from build123d import *

# Parameters (mm, degrees)
SKETCH1_R           = 12.5
SKETCH1_W           = 200
SKETCH1_H           = 15
BOSS_EXTRUDE1_DEPTH = 30
CUT_EXTRUDE2_REACH  = 204.793
SKETCH2_R           = 3.5
CUT_EXTRUDE3_START  = -27
SKETCH2_3_R         = 8
SKETCH2_3_R_2       = 3.5
CUT_EXTRUDE3_DEPTH  = 3
CUT_EXTRUDE4_REACH  = 204.793


with BuildPart() as part:
    # Sketch1 → Boss-Extrude1 (new body)
    with BuildSketch(Plane.XY):
        with Locations((175, 0)):
            Circle(SKETCH1_R)
        with Locations((100, 0)):
            Circle(SKETCH1_R)
        with Locations((100, 7.5)):
            Rectangle(SKETCH1_W, SKETCH1_H)
        with BuildLine():
            ThreePointArc((187.5, 0), (175, 12.5), (162.5, 0))
            Line((162.5, 0), (175, 0))
            Line((175, 0), (187.5, 0))
        make_face()
        with BuildLine():
            Line((175, 0), (162.5, 0))
            ThreePointArc((162.5, 0), (175, -12.5), (187.5, 0))
            Line((187.5, 0), (175, 0))
        make_face()
        with BuildLine():
            ThreePointArc((187.5, 0), (175, 12.5), (162.5, 0))
            Line((162.5, 0), (175, 0))
            Line((175, 0), (187.5, 0))
        make_face()
        with BuildLine():
            Line((175, 0), (162.5, 0))
            ThreePointArc((162.5, 0), (175, -12.5), (187.5, 0))
            Line((187.5, 0), (175, 0))
        make_face()
        with BuildLine():
            ThreePointArc((112.5, 0), (100, 12.5), (87.5, 0))
            Line((87.5, 0), (100, 0))
            Line((100, 0), (112.5, 0))
        make_face()
        with BuildLine():
            Line((100, 0), (87.5, 0))
            ThreePointArc((87.5, 0), (100, -12.5), (112.5, 0))
            Line((112.5, 0), (100, 0))
        make_face()
        with BuildLine():
            ThreePointArc((112.5, 0), (100, 12.5), (87.5, 0))
            Line((87.5, 0), (100, 0))
            Line((100, 0), (112.5, 0))
        make_face()
        with BuildLine():
            Line((100, 0), (87.5, 0))
            ThreePointArc((87.5, 0), (100, -12.5), (112.5, 0))
            Line((112.5, 0), (100, 0))
        make_face()
    extrude(amount=BOSS_EXTRUDE1_DEPTH)

    # Sketch2 → Cut-Extrude2 (cut, up to next)
    with BuildSketch(Plane.XY.offset(30), mode=Mode.PRIVATE) as cut_extrude2_sk1:
        with Locations((100, 0)):
            Circle(SKETCH2_R)
    cut_extrude2_tool1 = extrude(cut_extrude2_sk1.sketch, amount=-CUT_EXTRUDE2_REACH, mode=Mode.PRIVATE) & part.part
    # Sketch2 → Cut-Extrude2 (cut, up to next)
    with BuildSketch(Plane.XY.offset(30), mode=Mode.PRIVATE) as cut_extrude2_sk2:
        with Locations((175, 0)):
            Circle(SKETCH2_R)
    cut_extrude2_tool2 = extrude(cut_extrude2_sk2.sketch, amount=-CUT_EXTRUDE2_REACH, mode=Mode.PRIVATE) & part.part
    add(cut_extrude2_tool1.solids().sort_by_distance((100, 0, 30))[0], mode=Mode.SUBTRACT)
    add(cut_extrude2_tool2.solids().sort_by_distance((175, 0, 30))[0], mode=Mode.SUBTRACT)

    # Sketch2<3> → Cut-Extrude3 (cut)
    # profile 1 of 2: a face of its own
    with BuildSketch(Plane.XY.offset(30).offset(CUT_EXTRUDE3_START)):
        with Locations((100, 0)):
            Circle(SKETCH2_3_R)
        with Locations((100, 0)):
            Circle(SKETCH2_3_R_2, mode=Mode.SUBTRACT)
    # profile 2 of 2: a face of its own
    with BuildSketch(Plane.XY.offset(30).offset(CUT_EXTRUDE3_START)):
        with Locations((175, 0)):
            Circle(SKETCH2_3_R)
        with Locations((175, 0)):
            Circle(SKETCH2_3_R_2, mode=Mode.SUBTRACT)
    extrude(amount=-CUT_EXTRUDE3_DEPTH, mode=Mode.SUBTRACT)

    # Sketch3 → Cut-Extrude4 (cut, up to next)
    with BuildSketch(Plane.ZY, mode=Mode.PRIVATE) as cut_extrude4_sk1:
        with BuildLine():
            Line((0, 15), (30, 15))
            ThreePointArc((30, 15), (15, 8), (0, 15))
        make_face()
    cut_extrude4_tool1 = extrude(cut_extrude4_sk1.sketch, amount=-CUT_EXTRUDE4_REACH, mode=Mode.PRIVATE) & part.part
    add(cut_extrude4_tool1.solids().sort_by_distance((0, 12.152086, 15))[0], mode=Mode.SUBTRACT)


solid = part.part
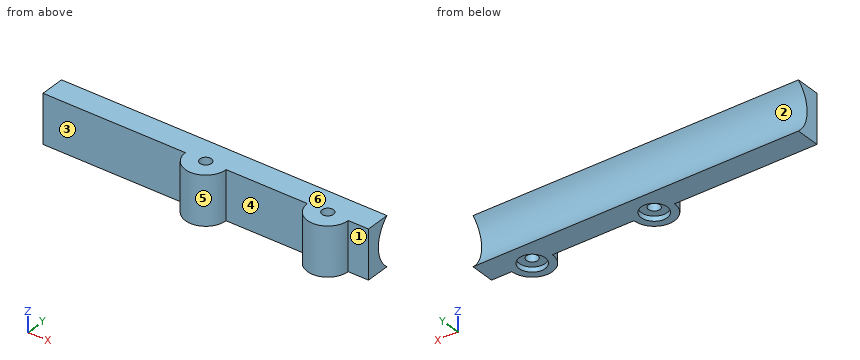
Can you work these out from the model? Positions are in its coordinate system, mm. Face numbers are marked on the shaded views. A direction names the side the tool comes from. Give positions to 0.01 mm unless a question says otherwise; leave off trailing zeros. Write each loop counter-clockwise with the first axis right and the second up, starting at its lowest first coordinate (ties: lowest second). Pieces come first, ordered by that corner, then holes. Notation, with made-up numbers: M 64.5,77 L 79.5,77 A11 cw 79.5,83 Z; hole C 54,70.25 d9. An arc over 180 degrees is marked long. Answer in a Markdown table with one row per item. Add a question column.
Item 1: For pin 1 Ø5 at (x, y) = (176.5, 1) entering from -Z; pin 2 Ø8 at (y, z) = (-5.5, 17.5) entering from +X; pin 3 Ø13 at (x, y) = (97.5, -2.5) entering from -Z; pin 4 Ø14 at (x, z) = (195, 12.5) entering from -Y, each with a flat end and sliding along its axis, tell me the tip position at first contact or that it passes through.
Item 2: We'd pull the mould along X, two halves only. Please class the marked faces 5 and 6: released by +X, released by -X, zero draft, split by the parting line, or undercut.
Item 3: Imagine slicing it at A-A, the plane z = 15. Write out the boundary of the cut face in (x, y), plus the area to 3 significant figures.
Item 4: Imagine slicing it at D-D, the plane x = 58.5. Write out the boundary of the cut face in (y, z).
Item 5: Imagine slicing it at B-B, the plane x = 175. Write out the boundary of the cut face in (y, z).
Item 6: Imagine slicing it at C-C, the plane y = -10.25. Write out the boundary of the cut face in (x, z), plus the area to 3 significant figures.
Item 7: Please list where these lines run through material, in increasing order: L1, parallel to Z at x = 179, y = -0.25; L2, parallel to X at y = -4, z = 4.25; L3, parallel to X at y = -8, z = 26.75.
Item 8: On a 3-axis mill with a long thin cutter (end or side, diameter ignored), from which of +Z, -Z, +X, -X, +Y, -Y can I reach the whole of each face in a straight line? I mean the marked faces 1, 2, 3 and 4. Say none if no direction works.
Evaluation:
| question | item | result |
|---|---|---|
| 1 | pin 1 | stops at z = 3 |
| 1 | pin 2 | stops at x = 187.41 |
| 1 | pin 3 | stops at z = 0 |
| 1 | pin 4 | stops at y = 0 |
| 2 | face 5 | undercut |
| 2 | face 6 | zero draft |
| 3 | outline | M 0,0 L 87.5,0 A12.5 ccw 112.5,0 L 162.5,0 A12.5 ccw 187.5,0 L 200,0 L 200,8 L 0,8 Z; hole C 100,0 d7; hole C 175,0 d7 |
| 3 | area | 2,010 mm² |
| 4 | outline | M 0,0 L 15,0 A19.57 cw 15,30 L 0,30 Z |
| 5 | outline | M -12.5,0 L -8,0 L -8,3 L -3.5,3 L -3.5,30 L -12.5,30 Z; M 3.5,3 L 8,3 L 8,0 L 15,0 A19.57 cw 15,30 L 3.5,30 Z |
| 6 | outline | M 92.85,0 L 107.15,0 L 107.15,30 L 92.85,30 Z; M 167.85,0 L 182.15,0 L 182.15,30 L 167.85,30 Z |
| 6 | area | 859 mm² |
| 7 | L1 | z = 3 to 30 |
| 7 | L2 | x = 88.16 to 111.84, 163.16 to 186.84 |
| 7 | L3 | x = 90.4 to 109.6, 165.4 to 184.6 |
| 8 | face 1 | +Z, -Z, +X, -Y |
| 8 | face 2 | +X, -X, +Y |
| 8 | face 3 | +Z, -Z, -X, -Y |
| 8 | face 4 | +Z, -Z, -Y |
